Input: part model. Units: mm. Frame: model coordinates. A direction names the side the tool comes from. Give positions to 0.01 mm unless a question says otherwise; leave off trailing zeros. Write each loop counter-clockwise with the first axis right and the second up, starting at its lowest first coordinate (ties: lowest second). Pieces come first, ordered by that corner, then holes. Notation, with made-up numbers: (50.25, -37.75) - (103.25, -37.75) arc R14 cw to (103.25, -32.75) - close; hole circle Ø10 at (-3, 41). An arc over 180 degrees is marked (long way). Use a Markdown table: item, result. Add a question column.
1. Section query A-A, the plane y = 85.5. Return loops of the section in (x, z), plus the area to 3 significant figures.
2. Mould query, pull axis Y, two halves, no side actions, for faces 1 (the cylindrical face through (-2, 83, -95)), 2 (the flat face through (-5, 86, 1)), 3 (the conical face through (12.774, 53.099, 0.351)), 4 (the flat face through (11, -90.5, 62)). Classes: released by +Y, released by -Y, zero draft, split by the parting line, or undercut.
3. Pin query (flat end, axial travel): pin 1 (7 mm diameter, centred on x = 8, y = -64.5, fed in from +Z); pin 2 (11.5 mm diameter, centred on x = 10.5, y = 24.5, fed in from -Z); pin 3 (3 mm diameter, centred on y = 87.5, z = 89, fed in from +X); pin 4 (4 mm diameter, centred on y = 85.5, z = -95, fed in from +X). Return the tip coordinate at first contact, or that it passes through.
4. Section query D-D, the plane x = -2.5. Return loops of the section in (y, z).
5. Section query C-C, the plane y = -60. Return loops of the section in (x, z), plus the area to 3 significant figures.
6. Material intervals for probe 1 along Y at (x, z) = (-1.1, -95); probe 2 along Y at (x, z) = (4.5, -51); probe 3 along X at (y, z) = (-17, -44), sorted ascending.
7. Set-up query: faces 5 (the flat face through (0, 86, -82)), 6 (the flat face through (23, 21, 30)), 7 (the flat face through (0, 86, 83)), 8 (the flat face through (0, 15, 1)), 9 (the flat face through (12, -62, 58)). Return all of +Z, -Z, +X, -X, +Y, -Y with unobstructed straight access to the full face (end or side cutting, diameter ignored); none if empty.
8. Section query B-B, the plane z = -95. Return loops of the section in (x, y), plus the area to 3 significant figures.
```python
from build123d import *

# Parameters (mm, degrees)
ESQUISSE1_W             = 130
ESQUISSE1_H             = 181
BASE_DEPTH              = 23
ESQUISSE2_W             = 116
ESQUISSE2_H             = 58
VIDE_CUBE_DEPTH         = 114.772799913
ESQUISSE3_R             = 29
VIDE_CYLINDRE_DEPTH     = 58
ESQUISSE5_W             = 5
ESQUISSE5_H             = 200
FIXATION_TIGE_DEPTH     = 10
ESQUISSE6_R             = 2.5
ENL_V_MAT_EXTRU_1_DEPTH = 137.818310178


with BuildPart() as part:
    # Esquisse1 → BASE (new body)
    with BuildSketch(Plane(origin=(0, 0, 0), x_dir=(0, 0, -1), z_dir=(1, 0, 0))):
        Rectangle(ESQUISSE1_W, ESQUISSE1_H)
    extrude(amount=BASE_DEPTH)

    # Esquisse2 → VIDE CUBE (cut, through all)
    with BuildSketch(Plane(origin=(23, 0, 0), x_dir=(0, 0, -1), z_dir=(1, 0, 0))):
        with Locations((0, -61.5)):
            Rectangle(ESQUISSE2_W, ESQUISSE2_H)
    extrude(amount=-VIDE_CUBE_DEPTH, mode=Mode.SUBTRACT)

    # Esquisse3 → VIDE CYLINDRE (cut)
    with BuildSketch(Plane.XZ.offset(32.5)):
        with Locations((33, 0)):
            Circle(ESQUISSE3_R)
    extrude(amount=-VIDE_CYLINDRE_DEPTH, mode=Mode.SUBTRACT)

    # Esquisse4 → VIDE CONE (revolve, cut)
    with BuildSketch(Plane(origin=(33, 0, 0), x_dir=(0, 0, -1), z_dir=(1, 0, 0))):
        Polygon((0, 25.5), (30.88316048, 25.5), (0, 105.5), align=None)
    revolve(axis=Axis((33, 105.5, 0), (0, -1, 0)), mode=Mode.SUBTRACT)

    # Esquisse5 → FIXATION TIGE (add)
    with BuildSketch(Plane(origin=(0, 90.5, 0), x_dir=(1, 0, 0), z_dir=(0, 1, 0))):
        with Locations((-2.5, 0)):
            Rectangle(ESQUISSE5_W, ESQUISSE5_H)
    extrude(amount=-FIXATION_TIGE_DEPTH)

    # Esquisse6 → Enl_v. mat.-Extru.1 (cut, through all)
    with BuildSketch(Plane(origin=(0, 0, 0), x_dir=(0, 0, -1), z_dir=(1, 0, 0))):
        with Locations((-95, 85.5)):
            Circle(ESQUISSE6_R)
        with Locations(Location((95, 85.5, 0), (0, 0, 180))):
            Circle(ESQUISSE6_R)
    extrude(amount=-ENL_V_MAT_EXTRU_1_DEPTH, mode=Mode.SUBTRACT)


solid = part.part
```
Result sheet:
| question | item | result |
|---|---|---|
| 1 | outline | (-5, -100) - (0, -100) - (0, -97.5) - (-5, -97.5) - close; (-5, -92.5) - (0, -92.5) - (0, -65) - (23, -65) - (23, 65) - (0, 65) - (0, 92.5) - (-5, 92.5) - close; (-5, 97.5) - (0, 97.5) - (0, 100) - (-5, 100) - close |
| 1 | area | 3,940 mm² |
| 2 | face 1 | undercut |
| 2 | face 2 | zero draft |
| 2 | face 3 | undercut |
| 2 | face 4 | released by -Y |
| 3 | pin 1 | stops at z = 65 |
| 3 | pin 2 | stops at z = -65 |
| 3 | pin 3 | stops at x = 0 |
| 3 | pin 4 | passes through |
| 4 | outline | (80.5, -100) - (90.5, -100) - (90.5, 100) - (80.5, 100) - close; hole circle Ø5 at (85.5, -95); hole circle Ø5 at (85.5, 95) |
| 5 | outline | (0, -65) - (23, -65) - (23, -58) - (0, -58) - close; (0, 58) - (23, 58) - (23, 65) - (0, 65) - close |
| 5 | area | 322 mm² |
| 6 | probe 1 | y = 80.5 to 83, 88 to 90.5 |
| 6 | probe 2 | y = -32.5 to 90.5 |
| 6 | probe 3 | x = 0 to 23 |
| 7 | face 5 | -Z, +X, +Y, -Y |
| 7 | face 6 | +Z, -Z, +X, +Y, -Y |
| 7 | face 7 | +Z, +X, +Y, -Y |
| 7 | face 8 | +Z, -Z, -X, -Y |
| 7 | face 9 | +X, -X, -Y |
| 8 | outline | (-5, 80.5) - (0, 80.5) - (0, 83) - (-5, 83) - close; (-5, 88) - (0, 88) - (0, 90.5) - (-5, 90.5) - close |
| 8 | area | 25.0 mm² |
